Part print with two shaded views. Sizes in mm from the minimum x, y, z corner. A direction names the side the tool comes from. Give positions to 0.01 mm unless a question says otherwise; leave off trailing zeros. Write each loop counter-clockwise with the first axis right and the second up, starting at its lowest first coordinate (ties: lowest second). Pieces come first, ordered by that corner, then holes. Notation, with made-up numbers: (-23, -25) -> (-8, -25) arc R17 cw to (-8, -17) -> close; hole circle Ø10 at (41, 78.25). An arc over 180 degrees is marked (long way). Write item = value, one per line. Start each with the question number.
Q1. Drop flat-ended pins along their axis: P1, Ø2.5, axis at x = 6.5, y = 5.5, coming from the -Z side; P2, Ø2, axis at x = 60, y = 11, coming from the +Z side (1 decimal); P3, Ø2.5, axis at x = 4, z = 13.5, coming from the +Y side. Give the stop position or say it passes through.
Q2. Saw through at A-A, the plane z = 9.25. Give the number of separate pieces and of enclosed holes in the cut face.
Q3. Tool access for the marked faces 4, 5 and 6: list every direction of +Z, -Z, +X, -X, +Y, -Y with a clear straight run to the whole face (end or side of a thin tool).
Q4. Wall check: line 1 (X direction, y = 5.5, z = 8.75) (1 decimal); line 2 (Y direction, x = 67.5, z = 7.75) (1 decimal); line 3 (Y direction, x = 67.5, z = 27.5) (1 decimal). Give the ranges that are in metal, low to high.
Q5. Mould opens along X. For the marked faces 1, 2 and 3 say: pulls with the +X half, pulls with the -X half, needs draft (parallel to the pull), parting line crosses it, or undercut.
Q6. Saw through at D-D, the plane z = 2.25. List the corners of the cut face in (x, y) (1 decimal).
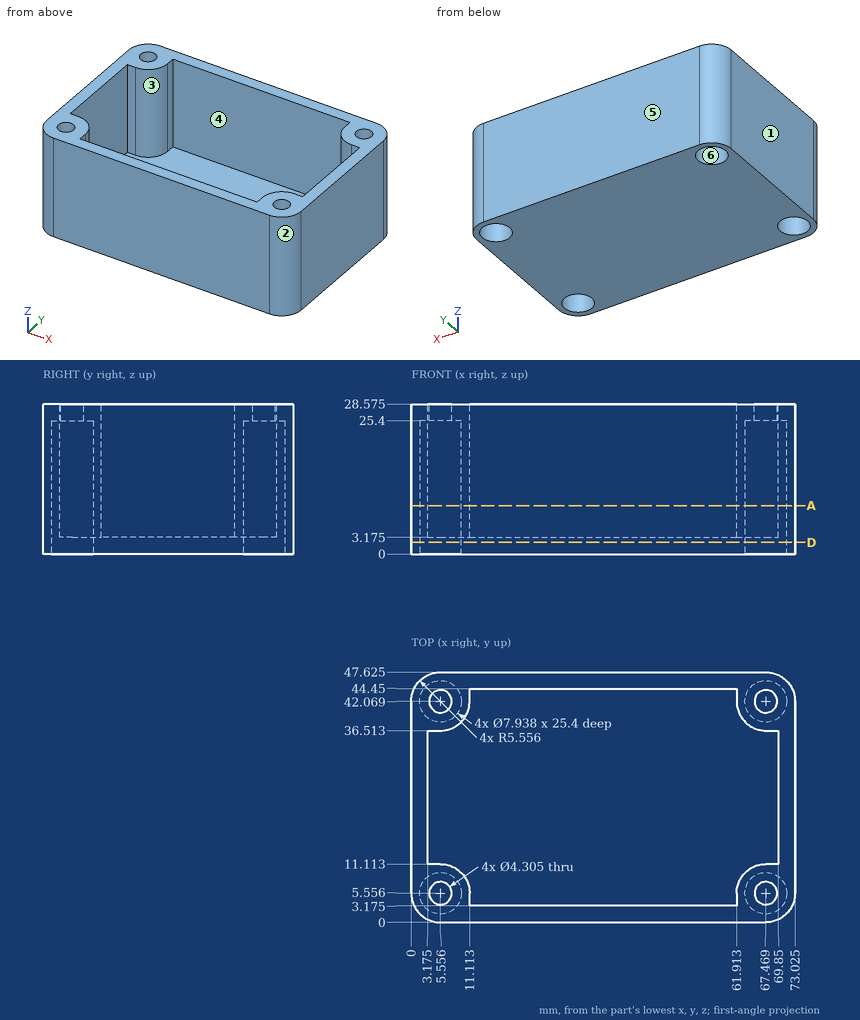
Report:
q1.P1 = 25.4
q1.P2 = 3.2
q1.P3 = 47.62
q2.separate_pieces = 1
q2.enclosed_holes = 5
q3.face_4 = +Z
q3.face_5 = +Z, -Z, +X, -X, +Y
q3.face_6 = -Z
q4.line_1 = 0 to 1.6, 9.5 to 11.1, 61.9 to 63.5, 71.4 to 73
q4.line_2 = 0 to 1.6, 9.5 to 11.1, 36.5 to 38.1, 46 to 47.6
q4.line_3 = 0 to 3.4, 7.7 to 11.1, 36.5 to 39.9, 44.2 to 47.6
q5.face_1 = pulls with the -X half
q5.face_2 = pulls with the +X half
q5.face_3 = undercut
q6.outline = (0, 5.6) arc R5.6 ccw to (5.6, 0) -> (67.5, 0) arc R5.6 ccw to (73, 5.6) -> (73, 42.1) arc R5.6 ccw to (67.5, 47.6) -> (5.6, 47.6) arc R5.6 ccw to (0, 42.1) -> close; hole circle Ø7.9 at (5.6, 5.6); hole circle Ø7.9 at (5.6, 42.1); hole circle Ø7.9 at (67.5, 5.6); hole circle Ø7.9 at (67.5, 42.1)
